Design review of the part built by this model. Coordinates are the model's own, in mm. A direction names the side the tool comes from. Give positions to 0.01 mm unless a question says otherwise; leave off trailing zeros. Loops run counter-clockwise (first coordinate to the right, second up) from the corner with the lowest first, then second, coordinate; pieces in that order, holes last. Notation, with made-up numbers: (55.5, 29) -> (97.5, 29) arc R10 cw to (97.5, 48) -> close; hole circle Ø6 at (-20, 35). An arc over 180 degrees is marked (long way). Answer in a Markdown table with one row per item. Add a question column.
(1) Consider section A-A on y = 8.75. Write out the cut boundary in (x, z), then the cut area to 3 significant figures.
(2) Consider section B-B on z = -153. Write out the cut boundary in (x, y), then the cut area to 3 significant figures.
(3) Consider section C-C on x = 97.5. Write out the cut boundary in (y, z), then the cut area to 4 significant figures.
(4) Consider section D-D on z = -52.5. Write out the cut boundary in (x, y).
(5) For pin 1 (2 mm diameter, centred on x = 41.5, z = -139, fed in from -Y); pin 2 (6 mm diameter, centred on y = 3, z = -129.5, fed in from +X); pin 3 (6 mm diameter, centred on y = 8.5, z = -46, fed in from -X), all flat-tipped, find the tip position at first contact; note any pin that passes through.
(6) For line 1 (Z direction, x = 4, y = 9.5); line 2 (X direction, y = 5.75, z = -161); line 3 (Z direction, x = 119, y = 7), list the stretches that pass through material, from the lowest coordinate up.
(7) Draft analysis for pull direction Z (two halves, no side actions). For faces 1 (the flat face through (0, 8, -4)), 2 (the flat face through (8, 10, -81)), 3 (the flat face through (62, 10, 0)), state which applies: +Z half, -Z half, draft (parallel to the pull), parting line (faces both ways), or undercut.
(8) For faces 4 (the flat face through (121, 8, -8)), 5 (the flat face through (4, 0, -159)), 6 (the flat face through (4, 8, -157)), 7 (the flat face through (8, 2, -161)), list the 3-axis set-ups (+Z, -Z, +X, -X, +Y, -Y) from which the entire face can be reached by the end or side of a thin tool; tool diameter is ignored.
Autodesk Inventor part; units mm, degrees
ref_plane "YZ Plane" through (0, 0, 0) normal (1, 0, 0) x (0, 1, 0)
ref_plane "XZ Plane" through (0, 0, 0) normal (0, 1, 0) x (-1, 0, 0)
ref_plane "XY Plane" through (0, 0, 0) normal (0, 0, 1) x (1, 0, 0)
sketch "Sketch1" plane through (0, 0, 0) normal (0, 1, 0) x (-1, 0, 0)
  line L0 (0, 0) -> (-125, 0)
  line L1 (-125, 0) -> (-125, -165)
  line L2 (-125, -165) -> (0, -165)
  line L3 (0, -165) -> (0, 0)
  circle A0 centre (-4, -4) radius 1.5
  circle A1 centre (-4, -161) radius 1.5
  circle A2 centre (-121, -4) radius 1.5
  circle A3 centre (-121, -161) radius 1.5
  line L4 (-125, 0) -> (-117, 0)
  line L5 (-117, 0) -> (-117, -8)
  line L6 (-117, -8) -> (-125, -8)
  line L7 (-125, -8) -> (-125, 0)
  line L8 (-125, -165) -> (-117, -165)
  line L9 (-117, -165) -> (-117, -157)
  line L10 (-117, -157) -> (-125, -157)
  line L11 (-125, -157) -> (-125, -165)
  line L12 (0, 0) -> (-8, 0)
  line L13 (-8, 0) -> (-8, -8)
  line L14 (-8, -8) -> (0, -8)
  line L15 (0, -8) -> (0, 0)
  line L16 (0, -165) -> (-8, -165)
  line L17 (-8, -165) -> (-8, -157)
  line L18 (-8, -157) -> (0, -157)
  line L19 (0, -157) -> (0, -165)
  line L20 (-117, -8) -> (-125, -8)
  line L21 (-125, -8) -> (-125, -157)
  line L22 (-125, -157) -> (-117, -157)
  line L23 (-117, -157) -> (-117, -8)
  line L24 (0, -8) -> (-8, -8)
  line L25 (-8, -8) -> (-8, -157)
  line L26 (-8, -157) -> (0, -157)
  line L27 (0, -157) -> (0, -8)
  dimension "d0" = 125
  dimension "d1" = 165
  dimension "d2" = 3
  dimension "d3" = 3
  dimension "d4" = 3
  dimension "d5" = 3
  dimension "d8" = 8
  dimension "d9" = 8
  dimension "d10" = 8
  dimension "d11" = 8
  dimension "d12" = 8
  dimension "d13" = 8
  dimension "d14" = 8
  dimension "d15" = 8
extrude "Extrusion1" add sketch "Sketch1" along normal blind 15.8 contours L3 L14 L13 L0 | L13 L25 L17 L2 L9 L23 L5 L0 | L5 L6 L1 L0 | L3 L2 L17 L18 | L9 L2 L1 L10
sketch "Sketch2" plane through (125, 0, -165) normal (0, 0, -1) x (-1, 0, 0)
  line L0 (8, 15.8) -> (0, 15.8)
  line L1 (8, 15.8) -> (117, 15.8)
  line L2 (117, 15.8) -> (117, 0.8)
  line L3 (117, 0.8) -> (8, 0.8)
  line L4 (8, 0.8) -> (8, 15.8)
  line L5 (0, 0) -> (125, 0)
  line L6 (8, 0.8) -> (117, 0.8)
  line L7 (117, 0.8) -> (117, 0)
  line L8 (117, 0) -> (8, 0)
  line L9 (8, 0) -> (8, 0.8)
  line L10 (8, 0.8) -> (68, 0.8)
  line L11 (68, 0.8) -> (68, 0)
  line L12 (68, 0) -> (8, 0)
  line L13 (8, 0) -> (8, 0.8)
  dimension "d16" = 109
  dimension "d17" = 15
  dimension "d18" = 60
  dimension "d19" = 0.8
extrude "Extrusion2" cut sketch "Sketch2" against normal blind 15 contours L3 L11 L5 L9
sketch "Sketch3" plane through (0, 0, 0) normal (0, -1, 0) x (1, 0, 0)
  line L0 (57, -150) -> (117, -150)
  line L1 (0, 0) -> (125, 0)
  line L2 (117, -150) -> (57, -150)
  line L3 (57, -150) -> (57, 0)
  line L4 (57, 0) -> (117, 0)
  line L5 (117, 0) -> (117, -150)
  line L6 (125, -165) -> (0, -165)
  line L7 (57, 0) -> (8, 0)
  line L8 (8, 0) -> (8, -165)
  line L9 (8, -165) -> (57, -165)
  line L10 (57, -165) -> (57, 0)
  line L11 (125, -165) -> (117, -165)
  line L12 (117, -165) -> (99.5, -165)
  line L13 (99.5, -165) -> (99.5, -150)
  line L14 (99.5, -150) -> (117, -150)
  line L15 (117, -150) -> (117, -165)
  dimension "d22" = 60
  dimension "d23" = 49
  dimension "d24" = 17.5
extrude "Extrusion3" cut sketch "Sketch3" against normal blind 3.8 contours L3 L1 L5 L0 | L10 L6 L8 L1 L3 | L0 L15 L6 L13
properties part number "7InchScreen"
Values follow:
| question | item | result |
|---|---|---|
| 1 | outline | (0, -165) -> (125, -165) -> (125, -157) -> (117, -157) -> (117, -8) -> (125, -8) -> (125, 0) -> (0, 0) -> (0, -8) -> (8, -8) -> (8, -157) -> (0, -157) -> close; hole circle Ø3 at (4, -161); hole circle Ø3 at (4, -4); hole circle Ø3 at (121, -161); hole circle Ø3 at (121, -4) |
| 1 | area | 18,200 mm2 |
| 2 | outline | (8, 3.8) -> (57, 3.8) -> (57, 0.8) -> (99.5, 0.8) -> (99.5, 3.8) -> (117, 3.8) -> (117, 15.8) -> (8, 15.8) -> close |
| 2 | area | 1,440 mm2 |
| 3 | outline | (0.8, -165) -> (15.8, -165) -> (15.8, 0) -> (3.8, 0) -> (3.8, -150) -> (0.8, -150) -> close |
| 3 | area | 2,025 mm2 |
| 4 | outline | (8, 3.8) -> (117, 3.8) -> (117, 15.8) -> (8, 15.8) -> close |
| 5 | pin 1 | y = 3.8 |
| 5 | pin 2 | x = 117 |
| 5 | pin 3 | x = 8 |
| 6 | line 1 | -165 to -162.5, -159.5 to -157, -8 to -5.5, -2.5 to 0 |
| 6 | line 2 | 0 to 2.5, 5.5 to 119.5, 122.5 to 125 |
| 6 | line 3 | -165 to -157, -8 to 0 |
| 7 | face 1 | draft |
| 7 | face 2 | undercut |
| 7 | face 3 | +Z half |
| 8 | face 4 | +X, +Y, -Y |
| 8 | face 5 | +Z, -Z, +X, -X, -Y |
| 8 | face 6 | -X, +Y, -Y |
| 8 | face 7 | +Z, -Z, -Y |
